Check sheet for the modelled part. Datum: model origin and axes. Units: mm. A direction names the side the tool comes from. Round coordinates to 2 decimals unless told otherwise and drop trailing zeros. Write each loop counter-clockwise with the first axis right and the second up, starting at its lowest first coordinate (ties: lowest second). Pieces come first, ordered by that corner, then holes. Notation, with made-up numbers: M -39,69 L 3,69 A8 ccw 3,81 Z; hole C 81,-21 d2. An arc over 180 degrees is marked long. Put each result on its own line as item: value.
```python
from build123d import *

# Parameters (mm, degrees)
ESQUISSE1_R        = 0.5
BOSS_EXTRU_4_DEPTH = 2


with BuildPart() as part:
    # Esquisse1 → Boss.-Extru.4 (new body)
    with BuildSketch(Plane(origin=(0, 0, 0), x_dir=(1, 0, 0), z_dir=(0, 1, 0))):
        with BuildLine():
            Line((-3.75, 15), (-2.471378864, 23.377208842))
            ThreePointArc((-2.471378864, 23.377208842), (0, 25.5), (2.471378864, 23.377208842))
            Line((2.471378864, 23.377208842), (3.75, 15))
            Line((3.75, 15), (3.75, -5))
            Line((3.75, -5), (-3.75, -5))
            Line((-3.75, -5), (-3.75, 15))
        make_face()
        with Locations(Location((0, 23, 0), (0, 0, 270))):
            Circle(ESQUISSE1_R, mode=Mode.SUBTRACT)
        with Locations(Location((0, 20, 0), (0, 0, 270))):
            Circle(ESQUISSE1_R, mode=Mode.SUBTRACT)
        with Locations(Location((0, 17, 0), (0, 0, 270))):
            Circle(ESQUISSE1_R, mode=Mode.SUBTRACT)
        with BuildLine():
            Line((-1.35, 0), (-1.35, 10))
            ThreePointArc((-1.35, 10), (0, 11.35), (1.35, 10))
            Line((1.35, 10), (1.35, 0))
            ThreePointArc((1.35, 0), (0, -1.35), (-1.35, 0))
        make_face(mode=Mode.SUBTRACT)
    extrude(amount=BOSS_EXTRU_4_DEPTH)


solid = part.part
```
1. Cross-section at A-A (z = -9.5). Enter the section's corners in (x, y).
Computed values:
outline: M -3.75,0 L -1.35,0 L -1.35,2 L -3.75,2 Z; M 1.35,0 L 3.75,0 L 3.75,2 L 1.35,2 Z
2. Scan lines: probe 1 along X at (y, z) = (0.2, -2.5); probe 2 along Z at (x, y) = (-0.75, 0.85); probe 3 along X at (y, z) = (1.2, -11). Record each from-to range of solid material in increasing order.
Computed values:
probe 1: x = -3.75 to -1.35, 1.35 to 3.75
probe 2: z = -25.38 to -11.12, 1.12 to 5
probe 3: x = -3.75 to -0.91, 0.91 to 3.75
3. Cross-section at C-C (y = 1.15). Enter the section's corners in (x, z), then the cut area to 3 significant figures.
Computed values:
outline: M -3.75,-15 L -2.47,-23.38 A2.5 ccw 2.47,-23.38 L 3.75,-15 L 3.75,5 L -3.75,5 Z; hole M -1.35,-10 A1.35 ccw 1.35,-10 L 1.35,0 A1.35 ccw -1.35,0 Z; hole C 0,-23 d1; hole C 0,-20 d1; hole C 0,-17 d1
area: 175 mm2
4. Cross-section at D-D (x = 2). Enter the section's corners in (y, z), then the cut area to 3 significant figures.
Computed values:
outline: M 0,-24.5 L 2,-24.5 L 2,5 L 0,5 Z
area: 59.0 mm2
5. Access from +Z, -Z, +X, -X, +Y, -Y to the whole of each face (thin tool, end or side, straight path). Record for faces 1 (the flat face through (0, 1, 5)), 2 (the cylindrical face through (0.03, 0.99, 1.35)).
Computed values:
face 1: +Z, +X, -X, +Y, -Y
face 2: +Y, -Y
6. Release check for a two-part mould opening along Z. For faces 3 (the flat face through (3.1, 0.99, -19.25)), 4 (the flat face through (3.75, 1, -5)), 5 (the cylindrical face through (-0.03, 0.99, -11.35)), 6 (the flat face through (1.35, 1, -5)) record: +Z half, -Z half, draft (parallel to the pull), parting line (faces both ways), or undercut.
Computed values:
face 3: -Z half
face 4: draft
face 5: undercut
face 6: undercut
7. Cross-section at B-B (x = -1). Enter the section's corners in (y, z).
Computed values:
outline: M 0,-25.29 L 2,-25.29 L 2,-10.91 L 0,-10.91 Z; M 0,0.91 L 2,0.91 L 2,5 L 0,5 Z
